```python
from build123d import *

# Parameters (mm, degrees)
SKETCH_1_R          = 3
EXTRUDE_1_DEPTH     = 64.8
SKETCH_2_R          = 6
EXTRUDE_2_DEPTH     = 1.5
SKETCH_10_R         = 1.5
CUT_EXTRUDE_1_DEPTH = 10


with BuildPart() as part:
    # 草图1 → 凸台-拉伸1 (new body)
    with BuildSketch(Plane.XY):
        Circle(SKETCH_1_R)
    extrude(amount=EXTRUDE_1_DEPTH)

    # 草图2 → 凸台-拉伸2 (add)
    with BuildSketch(Plane.XY.offset(17)):
        Circle(SKETCH_2_R)
    extrude(amount=-EXTRUDE_2_DEPTH)

    # 草图10 → 切除-拉伸1 (cut)
    with BuildSketch(Plane(origin=(0, -6.329883945, 9), x_dir=(-1, 0, 0), z_dir=(0, -1, 0))):
        with Locations(Location((0, 0, 0), (0, 0, 90))):
            Circle(SKETCH_10_R)
    extrude(amount=-CUT_EXTRUDE_1_DEPTH, mode=Mode.SUBTRACT)


solid = part.part
```
Can you work these out from the model? Positions are in its coordinate system, mm. A direction names the side the tool comes from. Give positions to 0.01 mm unless a question says otherwise; leave off trailing zeros. Order: outer loops, then holes, each group sorted by start corner. A loop starts at its lowest first (then second) coordinate and runs counter-clockwise, first axis right, second up. Notation, with made-up numbers: M 23,87 L 66,87 A24 cw 66,107 Z; hole C -35,-2.75 d1. An arc over 180 degrees is marked long. Write item = value, one per line. Start each with the question number.
Q1. I need wall thicknesses on probe 1 along Z at (x, y) = (0, -1); probe 2 along X at (y, z) = (-0.25, 9); probe 3 along Z at (x, y) = (1.5, 5.5). Which ranges of each line are inside material? Lowest first, please. Write a range as [from, to].
Q2. Suppose I cut it at C-C (z = 9). Write out the boundary of the cut face in (x, y), plus the area to 3 significant figures.
Q3. Will these pins go through, and if not, where does the flat tip stop? pin 1 Ø1 at (x, y) = (-4.5, 3) entering from +Z; pin 2 Ø1 at (x, z) = (-1, 44.5) entering from -Y; pin 3 Ø1.5 at (y, z) = (0.5, 34.5) entering from -X.
Q4. Suppose I cut it at D-D (z = 34.5). Write out the boundary of the cut face in (x, y), plus the area to 3 significant figures.
Q5. Suppose I cut it at A-A (x = 0). Write out the boundary of the cut face in (y, z).
Q6. We'd pull the mould along Z, two halves only. Please class faces 1 (the flat face through (0, 0, 64.8)), 2 (the flat face through (-3, -1, 15.5)), 3 (the cylindrical face through (-6, 0, 16)), 4 (the cylindrical face through (1.265, -0.042, 8.194)): pulls with the +Z half, pulls with the -Z half, needs draft (parallel to the pull), parting line crosses it, or undercut.
Q7. For faces 5 (the flat face through (0, 0, 0)), 6 (the cylindrical face through (1.384, -2.662, 7.642)), 7 (the cylindrical face through (-3, 0, 41)), which set-ups out of +Z, -Z, +X, -X, +Y, -Y let a thin tool reach every point of the face, with its end or its side?
Q8. Suppose I cut it at B-B (y = 0). Write out the boundary of the cut face in (x, z).
Check result:
q1.probe_1 = [0, 7.5], [10.5, 64.8]
q1.probe_2 = [-2.99, -1.5], [1.5, 2.99]
q1.probe_3 = [15.5, 17]
q2.outline = M -1.5,-2.6 L -1.5,2.6 A3 ccw Z; M 1.5,-2.6 A3 ccw 1.5,2.6 Z
q2.area = 11.1 mm2
q3.pin_1 = 17
q3.pin_2 = -2.96
q3.pin_3 = -3
q4.outline = C 0,0 d6
q4.area = 28.3 mm2
q5.outline = M -6,15.5 L -3,15.5 L -3,10.5 L 3,10.5 L 3,15.5 L 6,15.5 L 6,17 L 3,17 L 3,64.8 L -3,64.8 L -3,17 L -6,17 Z; M -3,0 L 3,0 L 3,7.5 L -3,7.5 Z
q6.face_1 = pulls with the +Z half
q6.face_2 = pulls with the -Z half
q6.face_3 = needs draft
q6.face_4 = undercut
q7.face_5 = -Z, +X, -X, +Y, -Y
q7.face_6 = -Z
q7.face_7 = +Z
q8.outline = M -6,15.5 L -3,15.5 L -3,0 L 3,0 L 3,15.5 L 6,15.5 L 6,17 L 3,17 L 3,64.8 L -3,64.8 L -3,17 L -6,17 Z; hole C 0,9 d3
